Could you check a few things on this model? Use its own coordinates, in mm. Face numbers are marked on the shaded views. A direction names the side the tool comes from. Round coordinates to 2 decimals unless told otherwise and drop trailing zeros. Write each loop counter-clockwise with the first axis right and the second up, starting at its lowest first coordinate (ties: lowest second). Pieces come first, ordered by that corner, then holes. Notation, with made-up numbers: (-31.5, 41) -> (20.5, 41) arc R27 ccw to (20.5, 75) -> close; hole circle Ø7 at (34, -11). An arc over 180 degrees is marked (long way). Answer in a Markdown table with one row per item.
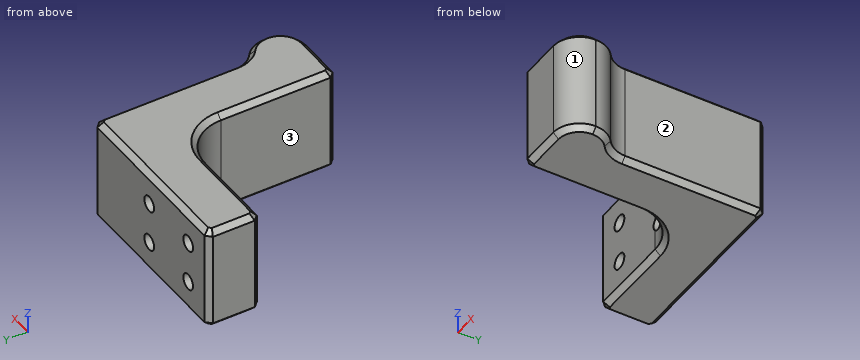
from build123d import *

# Parameters (mm, degrees)
EXTRUDE_3_DEPTH          = 20
FILLET_3_R               = 5
FILLET_4_R               = 5
FILLET_5_R               = 8
CUT_EXTRUDE_1_DEPTH      = 20
CUT_EXTRUDE_1_DEPTH_BACK = 20
SKETCH_6_R               = 1.5
CHAMFER_1_SIZE           = 1
CHAMFER_2_SIZE           = 1


with BuildPart() as part:
    # 草图5 → 凸台-拉伸3 (new body)
    with BuildSketch(Plane.XY):
        Polygon((-8.414313081, 8), (26.585686919, 8), (26.585686919, -22), (30.585686919, -22), (30.585686919, -32), (16.585686919, -32), (16.585686919, -2), (-8.414313081, -2), align=None)
    extrude(amount=EXTRUDE_3_DEPTH)

    # 圆角3
    # the kernel refuses this fillet: 5 mm, written as the material it takes off along each edge
    with BuildSketch(Plane(origin=(30.585686919, -32, -12.5), x_dir=(0, 1, 0), z_dir=(0, 0, 1))) as fillet_3_piece_1:
        with BuildLine():
            CenterArc((FILLET_3_R, FILLET_3_R), FILLET_3_R, 180, 90)
            Line((0, FILLET_3_R), (-FILLET_3_R * 0.02, FILLET_3_R))
            Line((-FILLET_3_R * 0.02, FILLET_3_R), (-FILLET_3_R * 0.02, -FILLET_3_R * 0.02))
            Line((-FILLET_3_R * 0.02, -FILLET_3_R * 0.02), (FILLET_3_R, -FILLET_3_R * 0.02))
            Line((FILLET_3_R, -FILLET_3_R * 0.02), (FILLET_3_R, 0))
        make_face()
    extrude(amount=45, mode=Mode.SUBTRACT)
    with BuildSketch(Plane(origin=(30.585686919, -22, -12.247448714), x_dir=(-1.0, -1.569411267609618e-12, 0), z_dir=(0, 0, 1))) as fillet_3_piece_2:
        with BuildLine():
            CenterArc((5, 4.898979486), FILLET_3_R, 180, 78.463040967)
            Line((0, 4.898979486), (-0.1, 4.898979486))
            Line((-0.1, 4.898979486), (-0.1, 0))
            Line((-0.1, 0), (0, -0.1))
            ThreePointArc((0, -0.1), (2, -0.1), (3.98, -0.09797959))
            Line((3.98, -0.09797959), (4, 0))
        make_face()
    extrude(amount=44.494897428, mode=Mode.SUBTRACT)

    # 圆角4
    fillet_4_edges = [part.edges().sort_by_distance(p)[0] for p in [
        (26.585686919, -22, 10),
    ]]
    fillet(fillet_4_edges, radius=FILLET_4_R)

    # 圆角5
    fillet_5_edges = [part.edges().sort_by_distance(p)[0] for p in [
        (16.585686919, -2, 10),
    ]]
    fillet(fillet_5_edges, radius=FILLET_5_R)

    # 草图6 → 切除-拉伸1 (cut, two sides: drawn at the far end of the back side and taken through both)
    with BuildSketch(Plane(origin=(0, -2, 0), x_dir=(-1, 0, 0), z_dir=(0, -1, 0)).offset(-CUT_EXTRUDE_1_DEPTH_BACK)):
        with Locations((2.414313081, -14)):
            Circle(SKETCH_6_R)
        with Locations((2.414313081, -6)):
            Circle(SKETCH_6_R)
        with Locations(Location((-9.585686919, -6, 0), (0, 0, 48.189685104))):
            Circle(SKETCH_6_R)
        with Locations(Location((-9.585686919, -14, 0), (0, 0, 48.189685104))):
            Circle(SKETCH_6_R)
    extrude(amount=CUT_EXTRUDE_1_DEPTH + CUT_EXTRUDE_1_DEPTH_BACK, mode=Mode.SUBTRACT)

    # 倒角1
    chamfer_1_edges = [part.edges().sort_by_distance(p)[0] for p in [
        (-8.414313081, 8, 10),
        (26.585686919, 8, 10),
        (16.585686919, -32, 10),
        (-8.414313081, -2, 10),
    ]]
    chamfer(chamfer_1_edges, length=CHAMFER_1_SIZE)

    # 倒角2
    chamfer_2_edges = [part.edges().sort_by_distance(p)[0] for p in [
        (30.585686919, -26.949489743, 0),
        (30.585686919, -26.949489743, 20),
        (29.121220825, -30.535533906, 0),
        (30.057822874, -24.662911508, 20),
        (29.121220825, -30.535533906, 20),
        (26.585686919, -5.949489743, 0),
        (26.585686919, -5.949489743, 20),
        (30.057822874, -24.662911508, 0),
        (27.113550964, -21.135047463, 0),
        (27.113550964, -21.135047463, 20),
        (16.585686919, -20.5, 0),
        (16.585686919, -20.5, 20),
        (14.242541169, -4.343145751, 0),
        (14.242541169, -4.343145751, 20),
        (9.085686919, 8, 0),
        (9.085686919, 8, 20),
        (21.585686919, -32, 0),
        (0.585686919, -2, 0),
        (-8.414313081, 3, 0),
        (17.085686919, -31.5, 0),
        (-7.914313081, -1.5, 0),
        (-7.914313081, 7.5, 0),
        (26.085686919, 7.5, 0),
        (21.585686919, -32, 20),
        (-8.414313081, 3, 20),
        (0.585686919, -2, 20),
        (17.085686919, -31.5, 20),
        (-7.914313081, -1.5, 20),
        (-7.914313081, 7.5, 20),
        (26.085686919, 7.5, 20),
    ]]
    chamfer(chamfer_2_edges, length=CHAMFER_2_SIZE)


solid = part.part
1) Imagine slicing it at A-A, the plane z = 6. Please give me the cut outline in (x, y), plus the area to 3 significant figures.
Findings:
| item | result |
|---|---|
| outline | (-8.41, -1) -> (-7.41, -2) -> (-3.91, -2) -> (-3.91, 8) -> (-7.41, 8) -> (-8.41, 7) -> close; (-0.91, -2) -> (8.09, -2) -> (8.09, 8) -> (-0.91, 8) -> close; (11.09, -2.4) arc R8 cw to (16.59, -10) -> (16.59, -31) -> (17.59, -32) -> (25.59, -32) arc R5 ccw to (30.59, -27) -> (30.59, -26.9) arc R5 ccw to (28.59, -22.9) arc R5 cw to (26.59, -18.9) -> (26.59, 7) -> (25.59, 8) -> (11.09, 8) -> close |
| area | 632 mm^2 |
2) Imagine slicing it at D-D, the plane y = -14. Please give me the cut outline in (x, z), plus the area to 3 significant figures.
Findings:
| item | result |
|---|---|
| outline | (16.59, 1) -> (17.59, 0) -> (25.59, 0) -> (26.59, 1) -> (26.59, 19) -> (25.59, 20) -> (17.59, 20) -> (16.59, 19) -> close |
| area | 198 mm^2 |
3) Please list where these lines run through material, in increasing order: line 1 (Z direction, x = 9, y = 5.5); line 2 (X direction, y = 2.5, z = 10); line 3 (Y direction, x = 6, z = 18.5).
Findings:
| item | result |
|---|---|
| line 1 | z = 0 to 4.62, 7.38 to 12.62, 15.38 to 20 |
| line 2 | x = -8.41 to 26.59 |
| line 3 | y = -2 to 8 |
4) Imagine slicing it at B-B, the plane x = 0.5. Please give me the cut outline in (y, z), plus the area to 3 significant figures.
Findings:
| item | result |
|---|---|
| outline | (-2, 1) -> (-1, 0) -> (7, 0) -> (8, 1) -> (8, 19) -> (7, 20) -> (-1, 20) -> (-2, 19) -> close |
| area | 198 mm^2 |
5) For the marked faces 1, 2 and 3, which set-ups out of +Z, -Z, +X, -X, +Y, -Y let a thin tool reach every point of the face, with its end or its side?
Findings:
| item | result |
|---|---|
| face 1 | +Z, -Z, +X, -Y |
| face 2 | +Z, -Z, +X, +Y |
| face 3 | +Z, -Z, -X, -Y |
6) For pin 1 (3.5 mm diameter, centred on x = 9.59, z = 14, fed in from +Y); pin 2 (2.5 mm diameter, centred on x = -2.41, z = 6, fed in from +Y); pin 3 (3.5 mm diameter, centred on x = 9.59, z = 6, fed in from -Y); pin 4 (8 mm diameter, centred on x = -2, z = 8, fed in from -Y), each with a flat end and sliding along its axis, tell me the tip position at first contact or that it passes through.
Findings:
| item | result |
|---|---|
| pin 1 | stops at y = 8 |
| pin 2 | passes through |
| pin 3 | stops at y = -2.49 |
| pin 4 | stops at y = -2 |
7) Imagine slicing it at C-C, the plane z = 10. Please give me the cut outline in (x, y), plus the area to 3 significant figures.
Findings:
| item | result |
|---|---|
| outline | (-8.41, -1) -> (-7.41, -2) -> (8.59, -2) arc R8 cw to (16.59, -10) -> (16.59, -31) -> (17.59, -32) -> (25.59, -32) arc R5 ccw to (30.59, -27) -> (30.59, -26.9) arc R5 ccw to (28.59, -22.9) arc R5 cw to (26.59, -18.9) -> (26.59, 7) -> (25.59, 8) -> (-7.41, 8) -> (-8.41, 7) -> close |
| area | 693 mm^2 |
